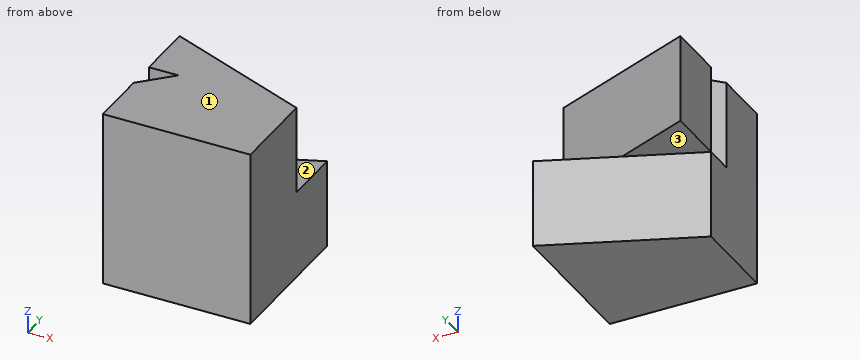
```python
from build123d import *

# Parameters (mm, degrees)
BOSS_EXTRUDE1_DEPTH = 15
BOSS_EXTRUDE2_DEPTH = 15
SKETCH6_W           = 25
SKETCH6_H           = 15
BOSS_EXTRUDE7_DEPTH = 15
BOSS_EXTRUDE8_DEPTH = 15


with BuildPart() as part:
    # Sketch1 → Boss-Extrude1 (new body)
    with BuildSketch(Plane.XY):
        Polygon((-25, 0), (0, 0), (0, 15), (-20, 15), (-25, 10), align=None)
    extrude(amount=BOSS_EXTRUDE1_DEPTH)

    # Sketch2 → Boss-Extrude2 (add)
    with BuildSketch(Plane(origin=(0, 0, 0), x_dir=(-1, 0, 0), z_dir=(0, 0, -1))):
        Polygon((25, 25), (25, 15), (0, 15), align=None)
    extrude(amount=-BOSS_EXTRUDE2_DEPTH)



with BuildPart() as body_2:
    # Sketch6 → Boss-Extrude7 (new body)
    with BuildSketch(Plane(origin=(0, 0, 0), x_dir=(-1, 0, 0), z_dir=(0, 0, -1))):
        with Locations((12.5, 7.5)):
            Rectangle(SKETCH6_W, SKETCH6_H)
    extrude(amount=BOSS_EXTRUDE7_DEPTH)


with BuildPart() as part_1:
    add(part.part)

    add(body_2.part)  # Boss-Extrude8 merges body 2
    # Sketch7 → Boss-Extrude8 (add)
    with BuildSketch(Plane(origin=(0, 0, 0), x_dir=(-1, 0, 0), z_dir=(0, 0, -1))):
        Polygon((0, 15), (0, 25), (25, 15), align=None)
    extrude(amount=BOSS_EXTRUDE8_DEPTH)


solid = part_1.part
```
Source: CAD feature listing. Evaluate the final solid. Frame: model axes, mm. Face numbers are marked on the shaded views. A direction names the side the tool comes from. Round coordinates to 2 decimals unless told otherwise and drop trailing zeros. Order: outer loops, then holes, each group sorted by start corner. A loop starts at its lowest first (then second) coordinate and runs counter-clockwise, first axis right, second up. Notation, with made-up numbers: (-24, 83) -> (31, 83) arc R19 ccw to (31, 115) -> close; hole circle Ø10 at (45, 37.5). An arc over 180 degrees is marked (long way). One line per item, written item: value. Start each with the question number.
Q1. Section query B-B (z = 1). Return the cut outline in (x, y).
Q2. Material intervals for probe 1 along Z at (x, y) = (-18.75, 18.5); probe 2 along Z at (x, y) = (-22.5, 12.75); probe 3 along Y at (x, z) = (-20.5, 4), sorted ascending.
Q3. Section query A-A (y = 17.5). Return the cut outline in (x, z).
Q4. Access query for the marked faces 1, 2 and 3. Directions: +Z, -Z, +X, -X, +Y, -Y. A direction counts if a zero-diameter tool reaches every point of the face in a straight line with its end or side. Return the directions, or none.
Q5. Section query C-C (x = -11.75). Return the cut outline in (y, z), plus the area to 3 significant figures.
Q6. Pin query (flat end, axial travel): pin 1 (1.5 mm diameter, centred on y = 21.5, z = 4.5, fed in from +X) (3 decimals). Return the tip coordinate at first contact, or that it passes through.
Q7. Section query D-D (y = 12.5). Return the cut outline in (x, z), plus the area to 4 significant figures.
Findings below:
1. outline: (-25, 0) -> (0, 0) -> (0, 15) -> (-25, 25) -> (-25, 15) -> (-20, 15) -> (-25, 10) -> close
2. probe 1: 0 to 15
2. probe 2: -15 to 0
2. probe 3: 0 to 14.5, 15 to 23.2
3. outline: (-25, 0) -> (-18.75, 0) -> (-18.75, -15) -> (0, -15) -> (0, 0) -> (-6.25, 0) -> (-6.25, 15) -> (-25, 15) -> close
4. face 1: +Z, +X, -X, +Y, -Y
4. face 2: +Z, +X, +Y
4. face 3: -Z, -X, +Y
5. outline: (0, -15) -> (20.3, -15) -> (20.3, 0) -> (19.7, 0) -> (19.7, 15) -> (0, 15) -> close
5. area: 600 mm²
6. pin 1: x = -14.375
7. outline: (-25, -15) -> (0, -15) -> (0, 15) -> (-22.5, 15) -> (-22.5, 0) -> (-25, 0) -> close
7. area: 712.5 mm²
